Geometry check sheet. Reference: the model listing, model coordinates, mm. Face numbers are marked on the shaded views. A direction names the side the tool comes from. Give positions to 0.01 mm unless a question says otherwise; leave off trailing zeros. Write each loop counter-clockwise with the first axis right and the second up, starting at its lowest first coordinate (ties: lowest second). Pieces come first, ordered by that corner, then holes. Notation, with made-up numbers: M 52,-3.5 L 95,-3.5 A7 ccw 95,0.5 Z; hole C 49.25,68.25 d10. An arc over 180 degrees is marked long. One line per item, written item: value. Start each with the question number.
1. Tool access check on the marked faces 4 and 5. Record the directions out of +Z, -Z, +X, -X, +Y, -Y that give a thin tool (end or side, any length) a straight path to the whole face; none if there is none.
2. Cross-section at D-D on x = 7.5. Record the cut outline in (y, z), then the cut area to 3 significant figures.
3. Cross-section at C-C on z = 9.25. Record the cut outline in (x, y).
4. Cross-section at B-B on y = 0.75. Record the cut outline in (x, z), then the cut area to 3 significant figures.
5. Cross-section at A-A on x = 0.5. Record the cut outline in (y, z), then the cut area to 3 significant figures.
6. Scan lines: line 1 (Y direction, x = 7, z = 9.75); line 2 (X direction, y = 7.5, z = 7.5); line 3 (X direction, y = 3.75, z = 9.75) (3 decimals). Record each from-to range of solid material in increasing order.
7. Release check for a two-part mould opening along Y. For the marked faces 1, 2 and 3 record: pulls with the +Y half, pulls with the -Y half, needs draft (parallel to the pull), parting line crosses it, or undercut.
from build123d import *

# Parameters (mm, degrees)
F0_W     = 10
F0_H     = 10
F1_DEPTH = 10
F3_DEPTH = 1
F5_DEPTH = 1
F7_DEPTH = 1


with BuildPart() as f1:
    # F0 (on Top) → F1 (new body)
    with BuildSketch(Plane.XY):
        with Locations((5, 5)):
            Rectangle(F0_W, F0_H)
    extrude(amount=F1_DEPTH)

    # F2 (on face) → F3 (cut)
    with BuildSketch(Plane.XZ):
        Polygon((4, 8), (2, 8), (4, 4), (4, 2), (6, 2), (6, 4), (8, 8), (6, 8), (5, 5.936254), align=None)
    extrude(amount=-F3_DEPTH, mode=Mode.SUBTRACT)

    # F4 (on face) → F5 (cut)
    with BuildSketch(Plane(origin=(0, 0, 0), x_dir=(0, -1, 0), z_dir=(-1, 0, 0))):
        Polygon((-6.5, 8.484827), (-8.5, 8.484827), (-6.5, 5), (-8.5, 1.56175), (-6.5, 1.56175), (-5, 3.56175), (-3.5, 1.56175), (-1.5, 1.56175), (-3.5, 5), (-1.5, 8.484827), (-3.5, 8.484827), (-5, 6.484827), align=None)
    extrude(amount=-F5_DEPTH, mode=Mode.SUBTRACT)

    # F6 (on face) → F7 (cut)
    with BuildSketch(Plane.XY.offset(10)):
        Polygon((8, 8), (2, 8), (2, 6.5), (6.5, 6.5), (2, 3.5), (2, 2), (8, 2), (8, 3.5), (3.5, 3.5), (8, 6.5), align=None)
    extrude(amount=-F7_DEPTH, mode=Mode.SUBTRACT)


solid = f1.part
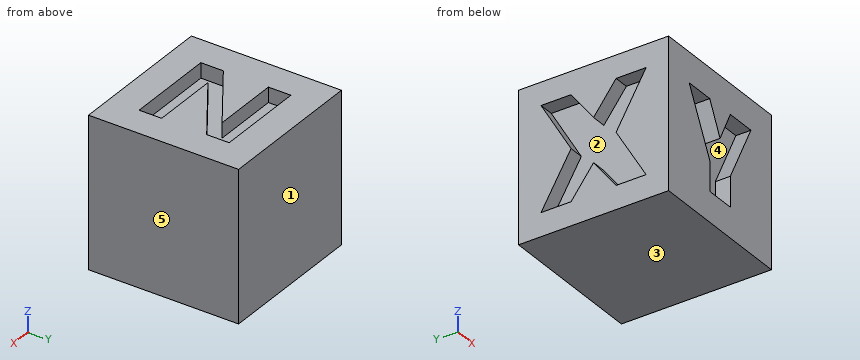
Report:
1. face 4: -Y
1. face 5: +Z, -Z, +X, +Y, -Y
2. outline: M 0,0 L 10,0 L 10,10 L 8,10 L 8,9 L 6.17,9 L 6.17,10 L 3.5,10 L 3.5,9 L 2,9 L 2,10 L 0,10 L 0,8 L 1,8 L 1,7 L 0,7 Z
2. area: 95.7 mm^2
3. outline: M 0,0 L 10,0 L 10,10 L 0,10 Z; hole M 2,2 L 8,2 L 8,3.5 L 3.5,3.5 L 8,6.5 L 8,8 L 2,8 L 2,6.5 L 6.5,6.5 L 2,3.5 Z
4. outline: M 0,0 L 10,0 L 10,10 L 0,10 Z; hole M 2,8 L 4,4 L 4,2 L 6,2 L 6,4 L 8,8 L 6,8 L 5,5.94 L 4,8 Z
4. area: 82.1 mm^2
5. outline: M 0,0 L 10,0 L 10,10 L 0,10 Z; hole M 1.5,1.56 L 3.5,1.56 L 5,3.56 L 6.5,1.56 L 8.5,1.56 L 6.5,5 L 8.5,8.48 L 6.5,8.48 L 5,6.48 L 3.5,8.48 L 1.5,8.48 L 3.5,5 Z
5. area: 71.4 mm^2
6. line 1: y = 0 to 2, 3.5 to 5.83, 8 to 10
6. line 2: x = 1 to 10
6. line 3: x = 0 to 2.375, 3.875 to 10
7. face 1: pulls with the +Y half
7. face 2: undercut
7. face 3: needs draft
